Can you work these out from the drawing? Everything is in mm from the part's minimum corner. A direction names the side the tool comes from. Round coordinates to 2 decimals unless told otherwise and drop trailing zeros. Write each loop counter-clockwise with the first axis right and the second up, starting at its lowest first coordinate (ties: lowest second). Pieces come first, ordered by that corner, then holes.
Q1. I'm going to push flat-ended pins straight in: pin 1 Ø10 at (x, z) = (149.5, 30) entering from -Y; pin 2 Ø9 at (x, y) = (94, 17.5) entering from -Z; pin 3 Ø2 at (x, z) = (87, 11.5) entering from +Y. Where does each tip first touch, or does it pass through?
Q2. If we section it at B-B (z = 10): Please give me the cut outline in (x, y).
Q3. If we section it at C-C (y = 9.5): Please give me the cut outline in (x, z).
Q4. For the marked faces 1 and 2, which set-ups out of +Z, -Z, +X, -X, +Y, -Y let a thin tool reach every point of the face, with its end or its side?
Q5. If we section it at D-D (z = 28.5): Please give me the cut outline in (x, y), plus the area to 3 significant figures.
Q6. Please list where these lines run through material, in increasing order: line 1 along Z through (x, y) = (157.5, 1.8); line 2 along Z through (x, y) = (155, 27); line 3 along Y through (x, z) = (160, 6.5).
Q7. If we section it at A-A (x = 32.5): Please give me the cut outline in (y, z), plus the area to 3 significant figures.
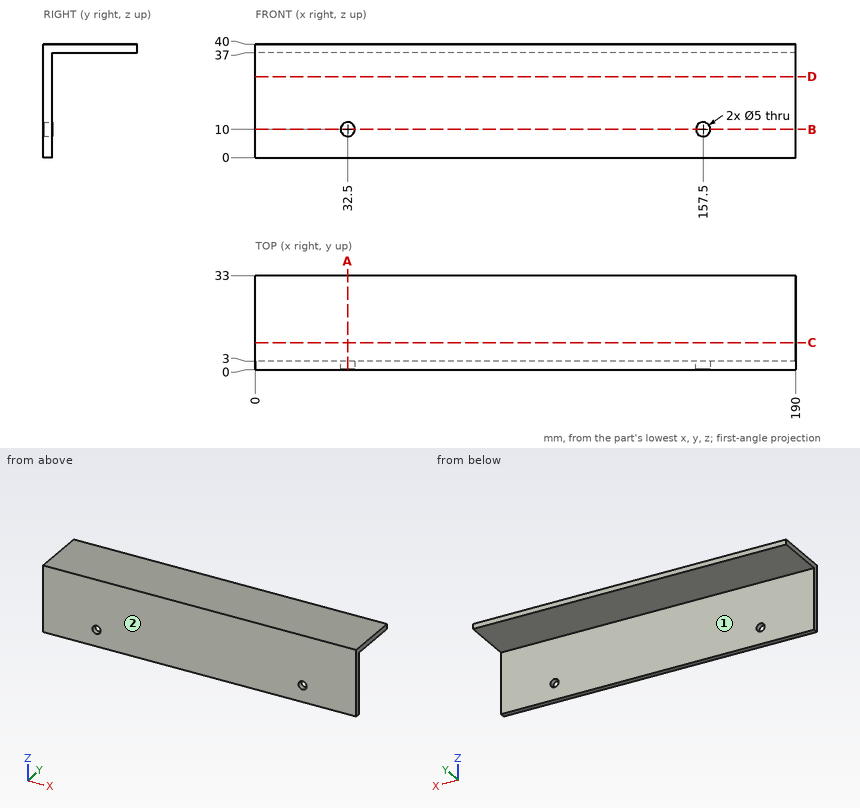
A:
1. pin 1: stops at y = 0
1. pin 2: stops at z = 37
1. pin 3: stops at y = 3
2. outline: (0, 0) - (30, 0) - (30, 3) - (0, 3) - close; (35, 0) - (155, 0) - (155, 3) - (35, 3) - close; (160, 0) - (190, 0) - (190, 3) - (160, 3) - close
3. outline: (0, 37) - (190, 37) - (190, 40) - (0, 40) - close
4. face 1: -Z, +X, -X, +Y
4. face 2: +Z, -Z, +X, -X, -Y
5. outline: (0, 0) - (190, 0) - (190, 3) - (0, 3) - close
5. area: 570 mm2
6. line 1: z = 0 to 7.5, 12.5 to 40
6. line 2: z = 37 to 40
6. line 3: y = 0 to 3
7. outline: (0, 0) - (3, 0) - (3, 7.5) - (0, 7.5) - close; (0, 12.5) - (3, 12.5) - (3, 37) - (33, 37) - (33, 40) - (0, 40) - close
7. area: 195 mm2
